Read the model definition and answer for the solid it produces. Units are mm, in the model's axes. A direction names the side the tool comes from. Give positions to 0.01 mm unless a question says otherwise; leave off trailing zeros. Order: outer loops, then holes, each group sorted by start corner. A loop starts at its lowest first (then second) coordinate and runs counter-clockwise, first axis right, second up. Notation, with made-up numbers: (11.5, 80) - (34.5, 80) arc R24 ccw to (34.5, 118) - close; hole circle Ø6 at (-9, 15). An arc over 180 degrees is marked (long way). Write each question's results on one line, items separated by ' | '.
Autodesk Inventor part; units mm, degrees
ref_plane "YZ Plane" through (0, 0, 0) normal (1, 0, 0) x (0, 1, 0)
ref_plane "XZ Plane" through (0, 0, 0) normal (0, 1, 0) x (-1, 0, 0)
ref_plane "XY Plane" through (0, 0, 0) normal (0, 0, 1) x (1, 0, 0)
sketch "Sketch1" plane through (0, 0, 0) normal (0, 0, 1) x (1, 0, 0)
  line L0 (-20, -10) -> (20, -10)
  line L1 (20, -10) -> (20, 10)
  line L2 (20, 10) -> (-20, 10)
  line L3 (-20, 10) -> (-20, -10)
  line L4 (-20, -10) -> (20, 10) construction
  line L5 (20, -10) -> (-20, 10) construction
  line L6 (-28, 0) -> (28, 0)
  circle A0 centre (-14, 0) radius 2.4
  circle A1 centre (14, 0) radius 2.4
  point P0 (0, 0)
  dimension "d0" = 40
  dimension "d1" = 20
  dimension "d2" = 4.8
  dimension "d3" = 4.8
  dimension "d4" = 6
  dimension "d5" = 6
extrude "Extrusion1" add sketch "Sketch1" along normal blind 8 contours L3 L6 A0 A1 L1 L0 | L3 L2 L1 L6 A1 A0
fillet "Fillet1" radius 2 4 edges at (20, -10, 4) (20, 10, 4) (-20, 10, 4) (-20, -10, 4)
sketch "Sketch2" plane through (0, 0, 8) normal (0, 0, 1) x (1, 0, 0)
  circle A0 centre (0, 0) radius 4.1
  circle A1 centre (0, 0) radius 6.1
  dimension "d9" = 8.2
  dimension "d24" = 2
extrude "Extrusion2" add sketch "Sketch2" along normal blind 10
chamfer "Chamfer1" distance 4 angle 45 1 edges at (-6.1, 0, 8)
chamfer "Chamfer2" distance 0.5 angle 45 1 edges at (-4.1, 0, 18)
sketch "Sketch5" plane through (0, 0, 8) normal (0, 0, 1) x (1, 0, 0)
  circle A0 centre (-14, 0) radius 2.4
  line L0 (-28, 0) -> (28, 0) construction
  line L1 (0, -14) -> (0, 14)
  circle A1 centre (-14, 0) radius 5
  circle A2 centre (14, 0) radius 2.4
  circle A3 centre (14, 0) radius 5
  point P0 (0, 0)
  dimension "d28" = 10
extrude "Extrusion4" cut sketch "Sketch5" along normal blind 8
sketch "Sketch6" plane through (0, 0, 8) normal (0, 0, 1) x (1, 0, 0)
  circle A0 centre (14, 0) radius 2.4
  circle A1 centre (-14, 0) radius 2.4
  circle A2 centre (14, 0) radius 5
  circle A3 centre (-14, 0) radius 5
  point P0 (0, 0)
  dimension "d31" = 10
  dimension "d32" = 10
extrude "Extrusion5" cut sketch "Sketch6" against normal blind 6
chamfer "Chamfer3" distance 0.5 angle 45 8 edges at (0, -10, 0) (19.4142, -9.4142, 0) (20, 0, 0) (19.4142, 9.4142, 0) (0, 10, 0) (-19.4142, 9.4142, 0) (-20, 0, 0) (-19.4142, -9.4142, 0)
equation "\"d3\" = d2"
equation "\"d5\" = d4"
equation "\"d32\" = d31"
properties part number "_3DPrint"
(1) Section D-D (z = 10.5) is taken. Give the vertices of the cut face in (x, y), plus the area to 3 significant figures.
Conclusion:
outline: circle Ø15.2 at (0, 0); hole circle Ø8.2 at (0, 0) | area: 129 mm^2
(2) Each of these flat-tipped pins is pushed along its axis until it touches: pin 1 (4 mm diameter, centred on x = 14, y = 0, fed in from +Z); pin 2 (6.5 mm diameter, centred on x = 0, y = 0, fed in from +Z); pin 3 (5 mm diameter, centred on x = 9.5, y = -0.5, fed in from +Z); pin 4 (4 mm diameter, centred on y = 2.5, z = 15, fed in from -X). Where does it stop, or does it pass through?
Conclusion:
pin 1: through | pin 2: z = 8 | pin 3: z = 11.09 | pin 4: x = -6.08
(3) The mould has two halves that part along X. Classify faces 3 (the face through (9, 0, 6)), 4 (the face through (5.866, 2.432, 11.75)), 5 (the face through (0, 0, 0)): pulls with the +X half, pulls with the -X half, needs draft (parallel to the pull), parting line crosses it, or undercut.
Conclusion:
face 3: undercut | face 4: parting line crosses it | face 5: needs draft
(4) Section A-A (x = -14) is taken. Give the vertices of the cut face in (y, z).
Conclusion:
outline: (-10, 0.5) - (-9.5, 0) - (-2.4, 0) - (-2.4, 2) - (-5, 2) - (-5, 8) - (-10, 8) - close; (2.4, 0) - (9.5, 0) - (10, 0.5) - (10, 8) - (5, 8) - (5, 2) - (2.4, 2) - close
(5) Section C-C (z = 1.5) is taken. Give the vertices of the cut face in (x, y), plus the area to 3 significant figures.
Conclusion:
outline: (-20, -8) arc R2 ccw to (-18, -10) - (18, -10) arc R2 ccw to (20, -8) - (20, 8) arc R2 ccw to (18, 10) - (-18, 10) arc R2 ccw to (-20, 8) - close; hole circle Ø4.8 at (-14, 0); hole circle Ø4.8 at (14, 0) | area: 760 mm^2
(6) Section B-B (y = 0) is taken. State how many separate pieces and enclosed holes the cut face has, plus the area to 3 significant figures.
Conclusion:
separate pieces: 3 | enclosed holes: 0 | area: 235 mm^2
(7) For faces 1 (the face through (-16.398, -0.106, 0.986)), 2 (the face through (0, 0, 8)), determine the directions among +Z, -Z, +X, -X, +Y, -Y from which every point of the face is accessible in a straight line to the end or side of a thin tool.
Conclusion:
face 1: +Z, -Z | face 2: +Z
(8) Consider probe 1 along X at (y, z) = (0, 5.5); probe 2 along X at (y, z) = (-4.25, 5.5); probe 3 along Y at (x, z) = (-14, 7). Determine where each line is inside the solid, lowest interval first. Write a range as [from, to].
Conclusion:
probe 1: [-20, -19], [-9, 9], [19, 20] | probe 2: [-20, -16.63], [-11.37, 11.37], [16.63, 20] | probe 3: [-10, -5], [5, 10]
